The figure shows three views and two pictorial views of one solid part (mm, origin at its lowest corner). Answer the questions. A direction names the side the tool comes from. Round coordinates to 2 decimals unless told otherwise and drop trailing zeros. Write each loop counter-clockwise with the first axis right and the second up, starting at its lowest first coordinate (ties: lowest second). Pieces come first, ordered by that corner, then holes. Notation, with made-up numbers: M 26.5,76 L 45.5,76 A18 ccw 45.5,86 Z; hole C -20,31 d6. An arc over 180 degrees is marked long. Answer in a Markdown table with one row per item.
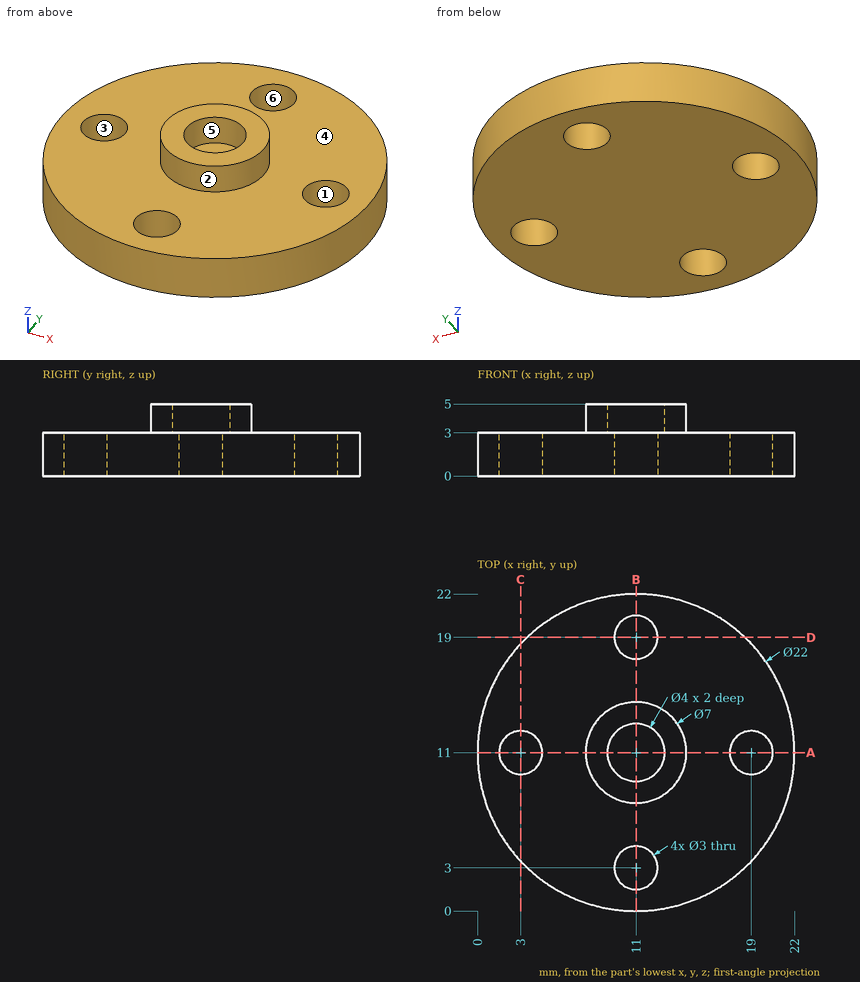
1. Given pin 1 (2.5 mm diameter, centred on x = 3, y = 11, fed in from +Z); pin 2 (2.5 mm diameter, centred on x = 11, y = 11, fed in from +Z); pin 3 (3 mm diameter, centred on y = 18.5, z = 4, fed in from +X); pin 4 (2 mm diameter, centred on x = 16, z = 1, fed in from +Y), each flat-ended and moving along its own axis, determine where each tip first touches the part or whether it passes through.
Calculated:
| item | result |
|---|---|
| pin 1 | passes through |
| pin 2 | stops at z = 3 |
| pin 3 | stops at x = 19.96 |
| pin 4 | stops at y = 21.25 |
2. Consider line 1 along Y through (x, z) = (11, 0.7); line 2 along Z through (x, y) = (20.25, 15.75); line 3 along Y through (x, z) = (18, 1.4). Determine where each line is inside the solid, lowest interval first. Write a range as from..to.
Calculated:
| item | result |
|---|---|
| line 1 | y = 0..1.5, 4.5..17.5, 20.5..22 |
| line 2 | z = 0..3 |
| line 3 | y = 2.51..9.88, 12.12..19.49 |
3. The part is cut by section A-A (y = 11). Determine the outline of the cut face in (x, z), plus the area to 3 significant figures.
Calculated:
| item | result |
|---|---|
| outline | M 0,0 L 1.5,0 L 1.5,3 L 0,3 Z; M 4.5,0 L 17.5,0 L 17.5,3 L 14.5,3 L 14.5,5 L 13,5 L 13,3 L 9,3 L 9,5 L 7.5,5 L 7.5,3 L 4.5,3 Z; M 20.5,0 L 22,0 L 22,3 L 20.5,3 Z |
| area | 54.0 mm² |
4. A tool of negligible diameter and unlimited length cuts with its end or side. For the marked faces 5 and 6, from which of +Z, -Z, +X, -X, +Y, -Y can it reach the whole face along a straight path? Write none if from no direction.
Calculated:
| item | result |
|---|---|
| face 5 | +Z |
| face 6 | +Z, -Z |
5. Determine the mould class of the marked faces 1, 2, 3 and 4 for opening direction X: released by +X, released by -X, zero draft, split by the parting line, or undercut.
Calculated:
| item | result |
|---|---|
| face 1 | undercut |
| face 2 | split by the parting line |
| face 3 | undercut |
| face 4 | zero draft |
6. The part is cut by section C-C (x = 3). Determine the outline of the cut face in (y, z).
Calculated:
| item | result |
|---|---|
| outline | M 3.45,0 L 9.5,0 L 9.5,3 L 3.45,3 Z; M 12.5,0 L 18.55,0 L 18.55,3 L 12.5,3 Z |
